Build history of the part. All positions in model axes, mm. Give positions to 0.01 mm unless a question says otherwise; leave off trailing zeros. Order: outer loops, then holes, each group sorted by start corner. A loop starts at its lowest first (then second) coordinate and runs counter-clockwise, first axis right, second up. Notation, with made-up numbers: (56, 48.25) -> (63, 48.25) arc R29 cw to (63, 68.25) -> close; hole circle Ø3 at (-39.5, -7.75). An arc over 180 degrees is marked (long way). Use a Markdown table: item, result. Add a question column.
```python
from build123d import *

# Parameters (mm, degrees)
F0_R     = 6.5
F0_R_2   = 1
F1_DEPTH = 1


with BuildPart() as f1:
    # F0 (on Top) → F1 (new body)
    with BuildSketch(Plane.XY):
        Circle(F0_R)
        with Locations((0, -4.618563)):
            Circle(F0_R_2, mode=Mode.SUBTRACT)
        with Locations((-4.618563, 0)):
            Circle(F0_R_2, mode=Mode.SUBTRACT)
        Circle(F0_R_2, mode=Mode.SUBTRACT)
        with Locations((4.618563, 0)):
            Circle(F0_R_2, mode=Mode.SUBTRACT)
        with Locations((0, 4.618563)):
            Circle(F0_R_2, mode=Mode.SUBTRACT)
    extrude(amount=F1_DEPTH)


solid = f1.part
```
(1) Band-saw the part on D-D on z = 0.5. Give the cut face in (x, y), plus the area to 3 significant figures.
(2) Mould opens along X. For faces 1 (the face through (-5.618, 0.044, 0.493)), 2 (the face through (-5.158, -3.955, 0.493)), 3 (the face through (-0.217, -0.976, 0.493)), 4 (the face through (1.4, 0.1, 0)) say: released by +X, released by -X, zero draft, split by the parting line, or undercut.
(3) Band-saw the part on C-C on y = 5. Give the cut face in (x, z), plus the area to 3 significant figures.
(4) Band-saw the part on A-A on y = 0. Give the cut face in (x, z).
(5) Wall check: probe 1 along Y at (x, z) = (0, 0.4); probe 2 along Y at (x, z) = (-0.25, 0.25); probe 3 along X at (y, z) = (4.75, 0.3). Give the ranges that are in metal, low to high.
Response:
| question | item | result |
|---|---|---|
| 1 | outline | circle Ø13 at (0, 0); hole circle Ø2 at (-4.62, 0); hole circle Ø2 at (0, -4.62); hole circle Ø2 at (0, 0); hole circle Ø2 at (0, 4.62); hole circle Ø2 at (4.62, 0) |
| 1 | area | 117 mm² |
| 2 | face 1 | undercut |
| 2 | face 2 | split by the parting line |
| 2 | face 3 | undercut |
| 2 | face 4 | zero draft |
| 3 | outline | (-4.15, 0) -> (-0.92, 0) -> (-0.92, 1) -> (-4.15, 1) -> close; (0.92, 0) -> (4.15, 0) -> (4.15, 1) -> (0.92, 1) -> close |
| 3 | area | 6.46 mm² |
| 4 | outline | (-6.5, 0) -> (-5.62, 0) -> (-5.62, 1) -> (-6.5, 1) -> close; (-3.62, 0) -> (-1, 0) -> (-1, 1) -> (-3.62, 1) -> close; (1, 0) -> (3.62, 0) -> (3.62, 1) -> (1, 1) -> close; (5.62, 0) -> (6.5, 0) -> (6.5, 1) -> (5.62, 1) -> close |
| 5 | probe 1 | y = -6.5 to -5.62, -3.62 to -1, 1 to 3.62, 5.62 to 6.5 |
| 5 | probe 2 | y = -6.5 to -5.59, -3.65 to -0.97, 0.97 to 3.65, 5.59 to 6.5 |
| 5 | probe 3 | x = -4.44 to -0.99, 0.99 to 4.44 |
